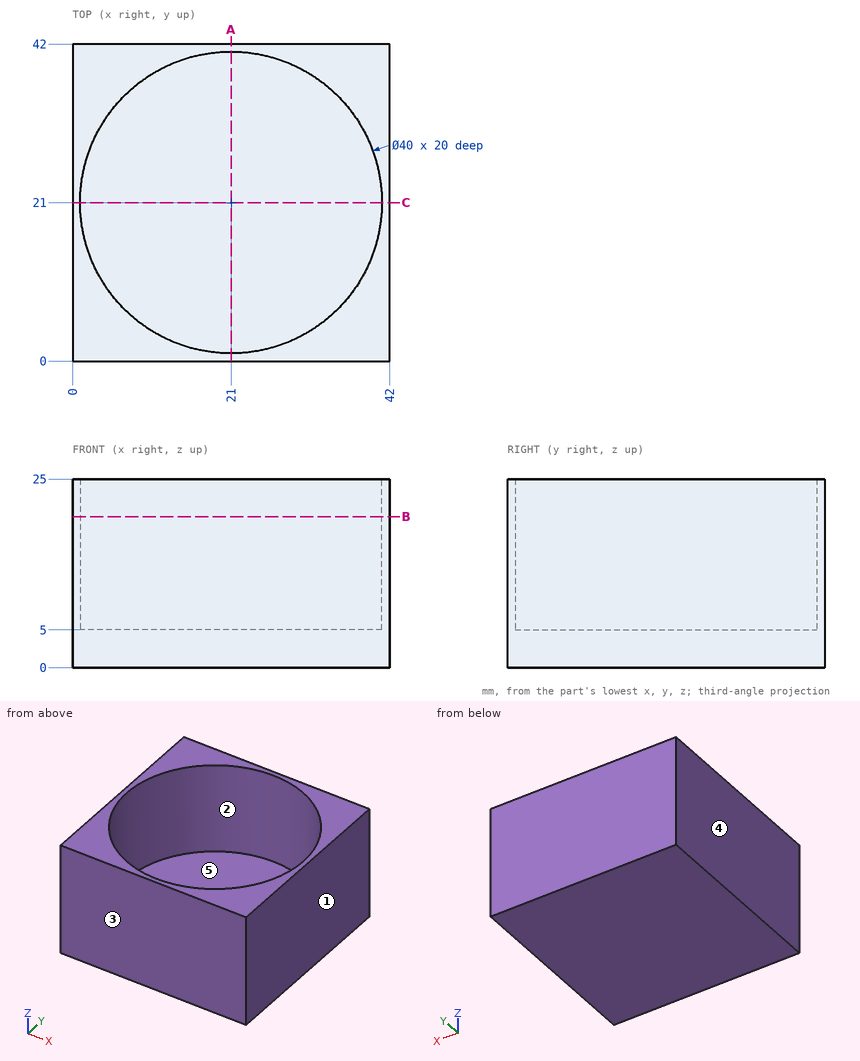
Here's the drawing with two shaded views (mm, measured from the low corner). I have some questions. A direction names the side the tool comes from. Round coordinates to 2 decimals unless told otherwise and drop trailing zeros. Loops run counter-clockwise (first coordinate to the right, second up) from the corner with the lowest first, then second, coordinate; pieces in that order, holes last. Notation, with made-up numbers: M -26.75,15.25 L 1.25,15.25 A24 cw 1.25,34.25 Z; hole C -27,54 d2. An arc over 180 degrees is marked long. Answer as a JSON object with one key per item and string values. Group by question number.
Q1. On a 3-axis mill with a long thin cutter (end or side, diameter ignored), from which of +Z, -Z, +X, -X, +Y, -Y can I reach the whole of each face in a straight line? I mean the marked faces 1 and 2. Say none if no direction works.
Q2. Will this pin go through, and if not, where does the flat tip stop? pin 1 (10 mm diameter, centred on x = 23, y = 18.5, fed in from +Z).
Q3. Imagine slicing it at B-B, the plane z = 20. Please give me the cut outline in (x, y), then the cut area to 3 significant figures.
Q4. We'd pull the mould along Y, two halves only. Please class the marked faces 3, 4 and 5: +Y half, -Y half, draft (parallel to the pull), parting line (faces both ways), or undercut.
Q5. Please list where these lines run through material, in increasing order: L1, parallel to Y at x = 21, z = 15.5; L2, parallel to Z at x = 29.5, y = 38.
Q6. Imagine slicing it at A-A, the plane x = 21. Please give me the cut outline in (y, z), then the cut area to 3 significant figures.
Findings:
{
 "1": {"face 1": "+Z, -Z, +X, +Y, -Y", "face 2": "+Z"},
 "2": {"pin 1": "stops at z = 5"},
 "3": {"outline": "M 0,0 L 42,0 L 42,42 L 0,42 Z; hole C 21,21 d40", "area": "507 mm2"},
 "4": {"face 3": "-Y half", "face 4": "draft", "face 5": "undercut"},
 "5": {"L1": "y = 0 to 1, 41 to 42", "L2": "z = 0 to 5"},
 "6": {"outline": "M 0,0 L 42,0 L 42,25 L 41,25 L 41,5 L 1,5 L 1,25 L 0,25 Z", "area": "250 mm2"}
}
